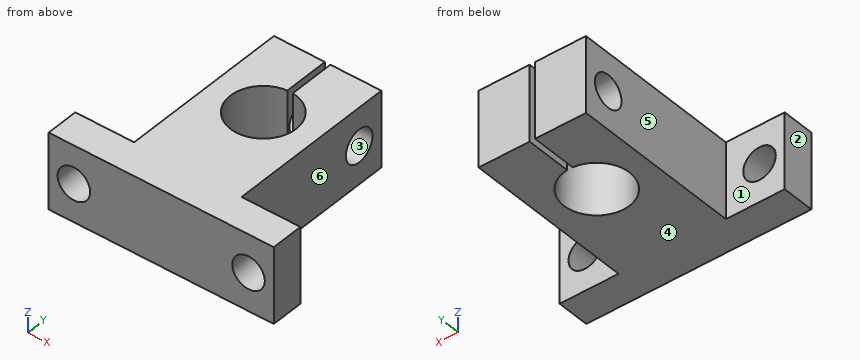
from build123d import *

# Parameters (mm, degrees)
Y_KSEKLIK_EKSTR_ZYON2_DEPTH = 14
IZIM3_R                     = 3
KES_EKSTR_ZYON1_DEPTH       = 30
IZIM4_R                     = 3
KES_EKSTR_ZYON2_DEPTH       = 41.234469053


with BuildPart() as part:
    # Çizim2 → Yükseklik-Ekstrüzyon2 (new body)
    with BuildSketch(Plane.XY):
        with BuildLine():
            Line((-0.504166667, 14.5), (-9.9, 14.5))
            Line((-9.9, 14.5), (-9.9, -17))
            Line((-9.9, -17), (-20.75, -17))
            Line((-20.75, -17), (-20.75, -23))
            Line((-20.75, -23), (20.75, -23))
            Line((20.75, -23), (20.75, -17))
            Line((20.75, -17), (9.9, -17))
            Line((9.9, -17), (9.9, 14.5))
            Line((9.9, 14.5), (0.504166667, 14.5))
            Line((0.504166667, 14.5), (0.504166667, 6.028956458))
            ThreePointArc((0.504166667, 6.028956458), (0, -6.05), (-0.504166667, 6.028956458))
            Line((-0.504166667, 6.028956458), (-0.504166667, 14.5))
        make_face()
    extrude(amount=-Y_KSEKLIK_EKSTR_ZYON2_DEPTH)

    # Çizim3 → Kes-Ekstrüzyon1 (cut)
    with BuildSketch(Plane.ZY.offset(9.9)):
        with Locations(Location((-7, 9.5, 0), (0, 0, 270))):
            Circle(IZIM3_R)
    extrude(amount=-KES_EKSTR_ZYON1_DEPTH, mode=Mode.SUBTRACT)

    # Çizim4 → Kes-Ekstrüzyon2 (cut, through all)
    with BuildSketch(Plane(origin=(0, -17, 0), x_dir=(1, 0, 0), z_dir=(0, 1, 0))):
        with Locations(Location((-16.1, 7, 0), (0, 0, 180))):
            Circle(IZIM4_R)
        with Locations((16.1, 7)):
            Circle(IZIM4_R)
    extrude(amount=-KES_EKSTR_ZYON2_DEPTH, mode=Mode.SUBTRACT)


solid = part.part
Geometry check sheet. Reference: the model listing, model coordinates, mm. Face numbers are marked on the shaded views. A direction names the side the tool comes from. Give positions to 0.01 mm unless a question says otherwise; leave off trailing zeros. Loops run counter-clockwise (first coordinate to the right, second up) from the corner with the lowest first, then second, coordinate; pieces in that order, holes last. Notation, with made-up numbers: (48, -10) -> (86, -10) arc R17 cw to (86, 20) -> close; hole circle Ø5 at (82.25, 56). An arc over 180 degrees is marked (long way). Answer in a Markdown table with one row per item. Add a question column.
1) Gauge pin test, flat ends, axial feed: P1, Ø8, axis at y = -10, z = -12.5, coming from the +X side; P2, Ø7, axis at x = -16.1, z = -7, coming from the +Y side; P3, Ø19.5, axis at x = 0, y = 0, coming from the -Z side; P4, Ø7, axis at y = 9.5, z = -7, coming from the -X side. Record the tip position at first contact, or that the pin passes through.
2) Draft check along Y on the marked faces 1, 2 and 3. Enter one of: pulls with the +Y half, pulls with the -Y half, needs draft (parallel to the pull), parting line crosses it, or undercut.
3) Material ranges on probe 1 along Y at (x, z) = (9, -7.25); probe 2 along Z at (x, y) = (16, -18); probe 3 along Y at (x, z) = (4, -9.25), recorded low to high. Write a range as from..to.
4) Cross-section at C-C on z = -7. Record the boundary of the cut face in (x, y).
5) Cross-section at A-A on y = 0. Record the boundary of the cut face in (x, z).
6) Cross-section at D-D on y = 9.5. Record the boundary of the cut face in (x, z).
7) Set-up check for the marked faces 4, 5 and 6: record each of +Z, -Z, +X, -X, +Y, -Y from which the full face is reachable in a straight line by a thin tool's end or side.
8) Cross-section at B-B on x = 16.1. Record the boundary of the cut face in (y, z), and give its area (3 significant figures).
Outcome:
| question | item | result |
|---|---|---|
| 1 | P1 | stops at x = 9.9 |
| 1 | P2 | stops at y = -17 |
| 1 | P3 | stops at z = -14 |
| 1 | P4 | stops at x = -9.9 |
| 2 | face 1 | pulls with the +Y half |
| 2 | face 2 | needs draft |
| 2 | face 3 | undercut |
| 3 | probe 1 | y = -23..6.51, 12.49..14.5 |
| 3 | probe 2 | z = -14..-10, -4..0 |
| 3 | probe 3 | y = -23..-4.54, 4.54..7.52, 11.48..14.5 |
| 4 | outline | (-20.75, -23) -> (-19.1, -23) -> (-19.1, -17) -> (-20.75, -17) -> close; (-13.1, -23) -> (13.1, -23) -> (13.1, -17) -> (9.9, -17) -> (9.9, 6.5) -> (0.5, 6.5) -> (0.5, 6.03) arc R6.05 cw (long way) to (-0.5, 6.03) -> (-0.5, 6.5) -> (-9.9, 6.5) -> (-9.9, -17) -> (-13.1, -17) -> close; (-9.9, 12.5) -> (-0.5, 12.5) -> (-0.5, 14.5) -> (-9.9, 14.5) -> close; (0.5, 12.5) -> (9.9, 12.5) -> (9.9, 14.5) -> (0.5, 14.5) -> close; (19.1, -23) -> (20.75, -23) -> (20.75, -17) -> (19.1, -17) -> close |
| 5 | outline | (-9.9, -14) -> (-6.05, -14) -> (-6.05, 0) -> (-9.9, 0) -> close; (6.05, -14) -> (9.9, -14) -> (9.9, 0) -> (6.05, 0) -> close |
| 6 | outline | (-9.9, -14) -> (-0.5, -14) -> (-0.5, -10) -> (-9.9, -10) -> close; (-9.9, -4) -> (-0.5, -4) -> (-0.5, 0) -> (-9.9, 0) -> close; (0.5, -14) -> (9.9, -14) -> (9.9, -10) -> (0.5, -10) -> close; (0.5, -4) -> (9.9, -4) -> (9.9, 0) -> (0.5, 0) -> close |
| 7 | face 4 | -Z, +X, -X, +Y, -Y |
| 7 | face 5 | +Z, -Z, -X, +Y |
| 7 | face 6 | +Z, -Z, +X, +Y |
| 8 | outline | (-23, -14) -> (-17, -14) -> (-17, -10) -> (-23, -10) -> close; (-23, -4) -> (-17, -4) -> (-17, 0) -> (-23, 0) -> close |
| 8 | area | 48.0 mm^2 |
